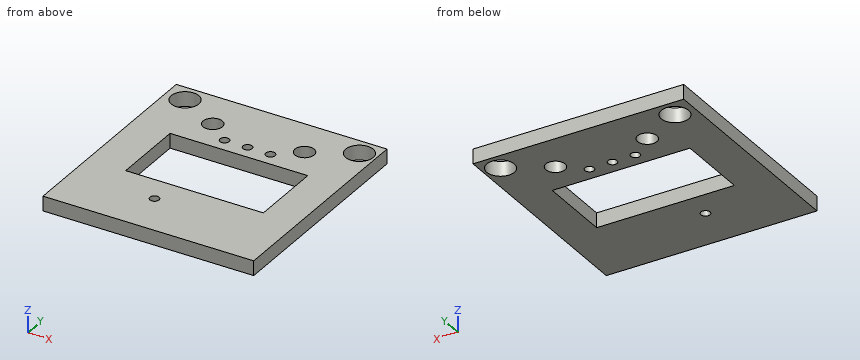
from build123d import *

# Parameters (mm, degrees)
F0_W     = 22.956962
F0_H     = 24
F0_R     = 0.5
F0_R_2   = 1.05
F1_DEPTH = 1.6
F2_W     = 15
F2_H     = 8
F3_DEPTH = 25
F4_R     = 1.5
F5_DEPTH = 25


with BuildPart() as f1:
    # F0 (on Top) → F1 (new body)
    with BuildSketch(Plane.XY):
        with Locations((-0.186301, 0)):
            Rectangle(F0_W, F0_H)
        with Locations((-2.54, -7)):
            Circle(F0_R, mode=Mode.SUBTRACT)
        with Locations((-2.5, 5.55)):
            Circle(F0_R, mode=Mode.SUBTRACT)
        with Locations((-5, 7.55)):
            Circle(F0_R_2, mode=Mode.SUBTRACT)
        with Locations((0, 5.55)):
            Circle(F0_R, mode=Mode.SUBTRACT)
        with Locations((2.5, 5.55)):
            Circle(F0_R, mode=Mode.SUBTRACT)
        with Locations((5, 7.55)):
            Circle(F0_R_2, mode=Mode.SUBTRACT)
    extrude(amount=-F1_DEPTH)

    # F2 (on face) → F3 (cut)
    with BuildSketch(Plane.XY):
        Rectangle(F2_W, F2_H)
    extrude(amount=-F3_DEPTH, mode=Mode.SUBTRACT)

    # F4 (on face) → F5 (cut)
    with BuildSketch(Plane.XY):
        with Locations((-9.5, 10)):
            Circle(F4_R)
        with Locations((9.5, 10)):
            Circle(F4_R)
    extrude(amount=-F5_DEPTH, mode=Mode.SUBTRACT)


solid = f1.part
The listing builds one solid part. Answer for the finished solid, in the listing's coordinates (mm). Round coordinates to 2 decimals unless told otherwise and drop trailing zeros. Write each loop counter-clockwise with the first axis right and the second up, starting at its lowest first coordinate (ties: lowest second). Pieces come first, ordered by that corner, then holes. Notation, with made-up numbers: (82.5, 31.25) - (103.5, 31.25) arc R17 cw to (103.5, 45.25) - close; hole circle Ø9 at (-13, -23). An arc over 180 degrees is marked (long way). Use one line per item in the form item = value. Start each with the question number.
Item 1: A cutting plane is placed at D-D (x = -5). Write down the section's boundary in (y, z).
Item 2: A cutting plane is placed at A-A (x = -9.5). Write down the section's boundary in (y, z).
Item 3: Find the intervals of material crossed by line 1 (X direction, y = 7.5, z = -1); line 2 (Y direction, x = -5, z = -0.3); line 3 (X direction, y = 3.75, z = -0.35), in increasing order. Write a range as [from, to].
Item 4: A cutting plane is placed at B-B (y = -1.75). Write down the section's boundary in (x, z), plus the area to 3 significant figures.
Item 5: A cutting plane is placed at C-C (z = -1). Give the number of separate pieces and of enclosed holes in the cut face, plus the area to 3 significant figures.
The answers:
q1.outline = (-12, -1.6) - (-4, -1.6) - (-4, 0) - (-12, 0) - close; (4, -1.6) - (6.5, -1.6) - (6.5, 0) - (4, 0) - close; (8.6, -1.6) - (12, -1.6) - (12, 0) - (8.6, 0) - close
q2.outline = (-12, -1.6) - (8.5, -1.6) - (8.5, 0) - (-12, 0) - close; (11.5, -1.6) - (12, -1.6) - (12, 0) - (11.5, 0) - close
q3.line_1 = [-11.66, -6.05], [-3.95, 3.95], [6.05, 11.29]
q3.line_2 = [-12, -4], [4, 6.5], [8.6, 12]
q3.line_3 = [-11.66, -7.5], [7.5, 11.29]
q4.outline = (-11.66, -1.6) - (-7.5, -1.6) - (-7.5, 0) - (-11.66, 0) - close; (7.5, -1.6) - (11.29, -1.6) - (11.29, 0) - (7.5, 0) - close
q4.area = 12.7 mm^2
q5.separate_pieces = 1
q5.enclosed_holes = 9
q5.area = 407 mm^2
